Here's how the part is built. I have some questions about the finished solid (model axes, mm). Face numbers are marked on the shaded views. A direction names the side the tool comes from. Round coordinates to 2 decimals unless told otherwise and drop trailing zeros. Loops run counter-clockwise (first coordinate to the right, second up) from the corner with the lowest first, then second, coordinate; pieces in that order, holes last. Notation, with made-up numbers: (30.25, 51.25) -> (54.25, 51.25) arc R31 cw to (54.25, 79.25) -> close; hole circle Ø8 at (80, -15). An arc over 180 degrees is marked (long way). Use one line per item in the form item = value. Start each with the question number.
Item 1: For the marked faces 4 and 5, which set-ups out of +Z, -Z, +X, -X, +Y, -Y let a thin tool reach every point of the face, with its end or its side?
Item 2: Thinking about a two-plate mould opening in X: for the marked faces 1, 2 and 3, which applies, released by +X, released by -X, zero draft, split by the parting line, or undercut?
Item 3: I'm going to push a flat-ended pin straight in: pin 1 Ø2 at (x, y) = (-1, -24) entering from +Z. Where does the tip first touch, or does it pass through?
Item 4: If I drill on L1, parallel to Z at x = 15.5, y = -10; L2, parallel to Y at x = -23, z = 35.5; L3, parallel to Y at x = -22, z = 48, over which ranges is the centre line in solid material (lowest first)? Write a range as [from, to].
Item 5: If we section it at C-C (x = 29): Write out the boundary of the cut face in (y, z).
Item 6: If we section it at B-B (z = 46): Write out the boundary of the cut face in (x, y) (3 decimals), then the cut area to 3 significant figures.
Item 7: If we section it at D-D (x = -19): Write out the boundary of the cut face in (y, z).
Item 8: If we section it at A-A (y = 0): Write out the boundary of the cut face in (x, z) (3 decimals), then the cut area to 3 significant figures.
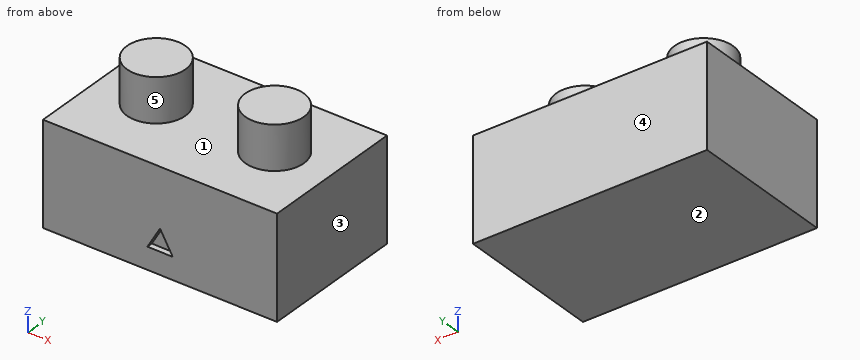
```python
from build123d import *

# Parameters (mm, degrees)
F0_W     = 80
F0_H     = 50
F1_DEPTH = 35
F3_DEPTH = 2
F4_R     = 10
F5_DEPTH = 15


with BuildPart() as f1:
    # F0 (on Top) → F1 (new body)
    with BuildSketch(Plane.XY):
        Rectangle(F0_W, F0_H)
    extrude(amount=F1_DEPTH)

    # F2 (on face) → F3 (cut)
    with BuildSketch(Plane.XZ.offset(25)):
        Polygon((0, 15), (-4.330127, 7.5), (4.330127, 7.5), align=None)
    extrude(amount=-F3_DEPTH, mode=Mode.SUBTRACT)

    # F4 (on face) → F5 (join)
    with BuildSketch(Plane.XY.offset(35)):
        with Locations((-20.077403, 0)):
            Circle(F4_R)
        with Locations((20.374997, 0)):
            Circle(F4_R)
    extrude(amount=F5_DEPTH)


solid = f1.part
```
Values found:
q1.face_4 = +Z, -Z, +X, -X, +Y
q1.face_5 = +Z
q2.face_1 = undercut
q2.face_2 = zero draft
q2.face_3 = released by +X
q3.pin_1 = 35
q4.L1 = [0, 35]
q4.L2 = [-9.56, 9.56]
q4.L3 = [-9.81, 9.81]
q5.outline = (-25, 0) -> (25, 0) -> (25, 35) -> (5.06, 35) -> (5.06, 50) -> (-5.06, 50) -> (-5.06, 35) -> (-25, 35) -> close
q6.outline = circle Ø20 at (-20.077, 0); circle Ø20 at (20.375, 0)
q6.area = 628 mm2
q7.outline = (-25, 0) -> (25, 0) -> (25, 35) -> (9.94, 35) -> (9.94, 50) -> (-9.94, 50) -> (-9.94, 35) -> (-25, 35) -> close
q8.outline = (-40, 0) -> (40, 0) -> (40, 35) -> (30.375, 35) -> (30.375, 50) -> (10.375, 50) -> (10.375, 35) -> (-10.077, 35) -> (-10.077, 50) -> (-30.077, 50) -> (-30.077, 35) -> (-40, 35) -> close
q8.area = 3,400 mm2
